Work out the finished part from the listing and answer in its coordinate system (mm). Round coordinates to 2 decimals unless told otherwise and drop trailing zeros. Loops run counter-clockwise (first coordinate to the right, second up) from the corner with the lowest first, then second, coordinate; pieces in that order, holes last. Notation, with made-up numbers: (33.5, -14.75) -> (82.5, -14.75) arc R28 cw to (82.5, 8.25) -> close; hole circle Ø6 at (33, 23). An arc over 180 degrees is marked (long way). Use one line per item in the form item = value.
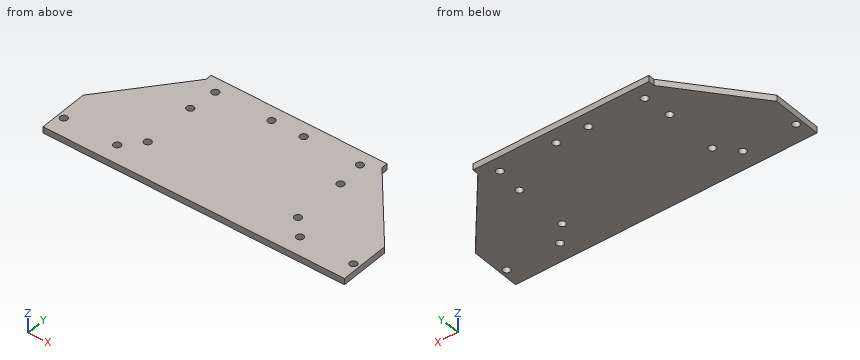
```python
from build123d import *

# Parameters (mm, degrees)
SKETCH1_W           = 88.9
SKETCH1_H           = 3.175
BOSS_EXTRUDE1_DEPTH = 51.435
SKETCH2_R           = 1.8288
CUT_EXTRUDE1_DEPTH  = 4.175
SKETCH3_R           = 1.8288
CUT_EXTRUDE2_DEPTH  = 4.175
BOSS_EXTRUDE2_DEPTH = 3.175
CUT_EXTRUDE3_DEPTH  = 4.175
SKETCH6_R           = 1.8288
CUT_EXTRUDE4_DEPTH  = 4.175


with BuildPart() as part:
    # Sketch1 → Boss-Extrude1 (new body)
    with BuildSketch(Plane(origin=(0, 0, 0), x_dir=(1, 0, 0), z_dir=(0, 1, 0))):
        Rectangle(SKETCH1_W, SKETCH1_H)
    extrude(amount=BOSS_EXTRUDE1_DEPTH)

    # Sketch2 → Cut-Extrude1 (cut, through all)
    with BuildSketch(Plane.XY.offset(1.5875)):
        with Locations((-36.576, 44.196)):
            Circle(SKETCH2_R)
        with Locations((-8.128, 44.196)):
            Circle(SKETCH2_R)
        with Locations((8.128, 44.196)):
            Circle(SKETCH2_R)
        with Locations((36.576, 44.196)):
            Circle(SKETCH2_R)
    extrude(amount=-CUT_EXTRUDE1_DEPTH, mode=Mode.SUBTRACT)

    # Sketch3 → Cut-Extrude2 (cut, through all)
    with BuildSketch(Plane.XY.offset(1.5875)):
        with Locations((-37.973, 3.175)):
            Circle(SKETCH3_R)
        with Locations((-37.973, 30.1244)):
            Circle(SKETCH3_R)
        with Locations((37.973, 3.175)):
            Circle(SKETCH3_R)
        with Locations((37.973, 30.1244)):
            Circle(SKETCH3_R)
    extrude(amount=-CUT_EXTRUDE2_DEPTH, mode=Mode.SUBTRACT)

    # Sketch4 → Boss-Extrude2 (add)
    with BuildSketch(Plane.XY.offset(1.5875)):
        Polygon((-44.45, 0), (-44.45, 48.26), (-76.2, 48.26), (-76.2, 0), (-76.2, -15.24), (76.2, -15.24), (76.2, 0), (76.2, 48.26), (44.45, 48.26), (44.45, 0), (0, 0), align=None)
    extrude(amount=-BOSS_EXTRUDE2_DEPTH)

    # Sketch5 → Cut-Extrude3 (cut, through all)
    with BuildSketch(Plane.XY.offset(1.5875)):
        Polygon((-76.2, 10.16), (-44.45, 48.26), (-76.2, 48.26), align=None)
        Polygon((44.45, 48.26), (76.2, 10.16), (76.2, 48.26), align=None)
    extrude(amount=-CUT_EXTRUDE3_DEPTH, mode=Mode.SUBTRACT)

    # Sketch6 → Cut-Extrude4 (cut, through all)
    with BuildSketch(Plane.XY.offset(1.5875)):
        with Locations((-73.1647, -5.842)):
            Circle(SKETCH6_R)
        with Locations((-46.2153, -5.842)):
            Circle(SKETCH6_R)
        with Locations((46.2153, -5.842)):
            Circle(SKETCH6_R)
        with Locations((73.1647, -5.842)):
            Circle(SKETCH6_R)
    extrude(amount=-CUT_EXTRUDE4_DEPTH, mode=Mode.SUBTRACT)


solid = part.part
```
(1) Consider L1, parallel to X at y = -4.5, z = 0.9; L2, parallel to X at y = 30, z = 0.15; L3, parallel to X at y = 45.5, z = 0.75. Determine where each line is inside the solid, lowest interval first.
Completed:
L1 = -76.2 to -74.41, -71.92 to -47.46, -44.97 to 44.97, 47.46 to 71.92, 74.41 to 76.2
L2 = -59.67 to -39.8, -36.15 to 36.15, 39.8 to 59.67
L3 = -46.75 to -37.86, -35.29 to -9.41, -6.85 to 6.85, 9.41 to 35.29, 37.86 to 46.75
(2) Find section C-C, the plane x = -62.5. Write down the section's boundary in (y, z).
Completed:
outline = (-15.24, -1.59) -> (26.6, -1.59) -> (26.6, 1.59) -> (-15.24, 1.59) -> close
(3) Find section D-D, the plane y = 16. Write down the section's boundary in (x, z).
Completed:
outline = (-71.33, -1.59) -> (71.33, -1.59) -> (71.33, 1.59) -> (-71.33, 1.59) -> close
(4) Given P1, Ø3.5, axis at x = -46.22, y = -5.84, coming from the +Z side; P2, Ø1, axis at y = 49, z = 0, coming from the +X side; P3, Ø1.6, axis at y = 49.5, z = 0.5, coming from the -X side, each flat-ended and moving along its own axis, determine where each tip first touches the part or whether it passes through.
Completed:
P1 = through
P2 = 44.45
P3 = -44.45
(5) Find section B-B, the plane z = 1. State how many separate pieces and enclosed holes the cut face has, then the cut area to 3 significant figures.
Completed:
separate_pieces = 1
enclosed_holes = 12
area = 8,620 mm2
(6) Find section A-A, the plane x = 8.5. Write down the section's boundary in (y, z) (1 decimal), then the cut area to 3 significant figures.
Completed:
outline = (-15.2, -1.6) -> (42.4, -1.6) -> (42.4, 1.6) -> (-15.2, 1.6) -> close; (46, -1.6) -> (51.4, -1.6) -> (51.4, 1.6) -> (46, 1.6) -> close
area = 200 mm2
